Design review of the part built by this model. Coordinates are the model's own, in mm. Face numbers are marked on the shaded views. A direction names the side the tool comes from. Coordinates: 2 decimals unless noted, no trailing zeros. Write each loop counter-clockwise with the first axis right and the second up, starting at its lowest first coordinate (ties: lowest second). Pieces come first, ordered by that corner, then holes. Notation, with made-up numbers: M 33.5,37.5 L 46.5,37.5 A21 ccw 46.5,53.5 Z; hole C 89.5,74 d8. An arc over 180 degrees is marked long. Return JSON: item names as keys, results as strings. Group by question number.
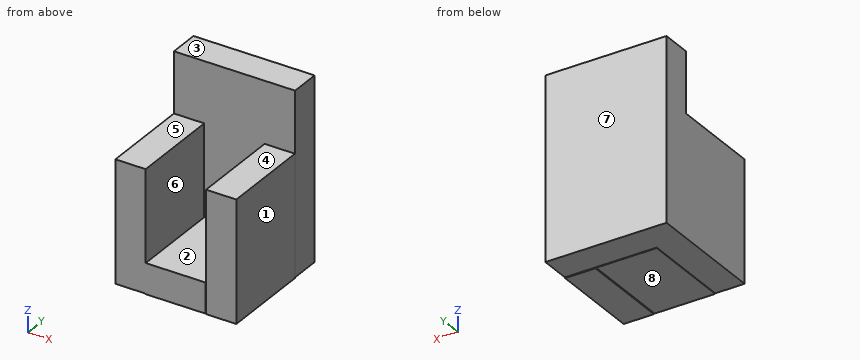
```python
from build123d import *

# Parameters (mm, degrees)
F1_DEPTH = 50.8
F0_W     = 38.1
F0_H     = 50.8
F2_DEPTH = 12.7
F3_W     = 25.4
F3_H     = 12.7
F4_DEPTH = 38.1
F5_W     = 12.7
F5_H     = 50.8
F6_DEPTH = 38.1


with BuildPart() as f1:
    # F0 (on Right) → F1 (new body)
    with BuildSketch(Plane.YZ):
        Polygon((38.1, 0), (38.1, -25.4), (38.1, -76.2), (50.8, -76.2), (50.8, 0), align=None)
    extrude(amount=F1_DEPTH)

    # F0 (on Right) → F2 (join)
    with BuildSketch(Plane.YZ):
        with Locations((19.05, -50.8)):
            Rectangle(F0_W, F0_H)
    extrude(amount=F2_DEPTH)

    # F3 (on Front) → F4 (join)
    with BuildSketch(Plane.XZ):
        with Locations((25.014978, -70.070165)):
            Rectangle(F3_W, F3_H)
    extrude(amount=-F4_DEPTH)

    # F5 (on Front) → F6 (join)
    with BuildSketch(Plane.XZ):
        with Locations((44.36385, -51.16912)):
            Rectangle(F5_W, F5_H)
    extrude(amount=-F6_DEPTH)


solid = f1.part
```
Item 1: Add section B-B (z = -37.5). Write out the cut boundary in (x, y).
Item 2: The part is to be moulded in two halves that separate along X. For the marked faces 1, 2 and 3, say which applies: pulls with the +X half, pulls with the -X half, needs draft (parallel to the pull), parting line crosses it, or undercut.
Item 3: Machinability: for the marked faces 4, 5, 6, 7 and 8, which of the approach directions +Z, -Z, +X, -X, +Y, -Y give a long, thin tool a straight path to every point of the face, cutting with its end or side? Answer none if there is none.
Item 4: Add section C-C (x = 45). Write out the cut boundary in (y, z), plus the area to 3 significant figures.
Item 5: Add section A-A (y = 37). Write out the cut boundary in (x, z), plus the area to 3 significant figures.
Item 6: Add section D-D (x = 34). Write out the cut boundary in (y, z).
Item 7: For line 1 (X direction, y = 4.5, z = -61.5); line 2 (X direction, y = 36, z = -68); line 3 (Y direction, x = 35, z = -35.5), list the stretches that pass through material, from the lowest coordinate up.
Item 8: For pin 1 (4 mm diameter, centred on x = 21.5, z = -35, fed in from -Y); pin 2 (10 mm diameter, centred on y = 15, z = -67.5, fed in from +X); pin 3 (15 mm diameter, centred on x = 28, y = 30.5, fed in from -Z), all flat-tipped, find the tip position at first contact; note any pin that passes through.
Geometry check:
{
 "1": {"outline": "M 0,0 L 12.7,0 L 12.7,38.1 L 38.01,38.1 L 38.01,0 L 50.71,0 L 50.71,38.1 L 50.8,38.1 L 50.8,50.8 L 0,50.8 Z"},
 "2": {"face 1": "pulls with the +X half", "face 2": "undercut", "face 3": "needs draft"},
 "3": {"face 4": "+Z, +X, -Y", "face 5": "+Z, +X, -X, -Y", "face 6": "+Z, -Y", "face 7": "+Z, -Z, +X, -X, +Y", "face 8": "-Z, -X, +Y, -Y"},
 "4": {"outline": "M 0,-76.57 L 38.1,-76.57 L 38.1,-76.2 L 50.8,-76.2 L 50.8,0 L 38.1,0 L 38.1,-25.77 L 0,-25.77 Z", "area": "2,900 mm^2"},
 "5": {"outline": "M 0,-76.2 L 12.31,-76.2 L 12.31,-76.42 L 37.71,-76.42 L 37.71,-63.72 L 12.7,-63.72 L 12.7,-25.4 L 0,-25.4 Z; M 38.01,-76.57 L 50.71,-76.57 L 50.71,-25.77 L 38.01,-25.77 Z", "area": "1,610 mm^2"},
 "6": {"outline": "M 0,-76.42 L 38.1,-76.42 L 38.1,-76.2 L 50.8,-76.2 L 50.8,0 L 38.1,0 L 38.1,-63.72 L 0,-63.72 Z"},
 "7": {"line 1": "0 to 12.7, 38.01 to 50.71", "line 2": "0 to 37.71, 38.01 to 50.71", "line 3": "38.1 to 50.8"},
 "8": {"pin 1": "y = 38.1", "pin 2": "x = 50.71", "pin 3": "z = -76.42"}
}
